The listing builds one solid part. Answer for the finished solid, in the listing's coordinates (mm). Give positions to 0.01 mm unless a question says otherwise; leave off trailing zeros. Loops run counter-clockwise (first coordinate to the right, second up) from the corner with the lowest first, then second, coordinate; pieces in that order, holes last. Notation, with made-up numbers: M 5,64.5 L 51,64.5 A20 cw 51,87.5 Z; hole C 2.5,-14.5 d4. An arc over 180 degrees is marked long. Use one line per item in the form item = value. Start each with the question number.
1. Straight lines are drawn through the part: line 1 (X direction, y = 1.45, z = 49); line 2 (X direction, y = 0.2, z = -42). For each, find the intervals that lie inside material, in ascending order. Write a range as from..to.
2. The part is cut by section C-C (z = 41.5). Write down the section's boundary in (x, y), and give its area (3 significant figures).
3. The part is cut by section A-A (y = 0.6). Give the number of separate pieces and of enclosed holes in the cut face, and give its area (3 significant figures).
4. The part is cut by section B-B (z = -44). Write down the section's boundary in (x, y), and give its area (4 significant figures).
5. The mould has two halves that part along X. Classify faces 1 (the face through (49.9, 0.7, -47.6)), 2 (the face through (-1, 1.5, -1)), 3 (the face through (-49.9, 0.7, -47.6)), 4 (the face through (-52.98, 0.76, 23.67)): released by +X, released by -X, zero draft, split by the parting line, or undercut.
from build123d import *

# Parameters (mm, degrees)
SKETCH1_W           = 115
SKETCH1_H           = 110
BOSS_EXTRUDE1_DEPTH = 1.5
CHAMFER1_SIZE       = 15
SKETCH3_R           = 1.5
CUT_EXTRUDE1_DEPTH  = 1.5
SKETCH4_R           = 1.5
CUT_EXTRUDE2_DEPTH  = 1.5


with BuildPart() as part:
    # Sketch1 → Boss-Extrude1 (new body)
    with BuildSketch(Plane(origin=(0, 0, 0), x_dir=(1, 0, 0), z_dir=(0, 1, 0))):
        Rectangle(SKETCH1_W, SKETCH1_H)
    extrude(amount=BOSS_EXTRUDE1_DEPTH)

    # Chamfer1
    chamfer1_edges = [part.edges().sort_by_distance(p)[0] for p in [
        (57.5, 0.75, 55),
        (-57.5, 0.75, 55),
        (-57.5, 0.75, -55),
        (57.5, 0.75, -55),
    ]]
    chamfer(chamfer1_edges, length=CHAMFER1_SIZE)

    # Sketch3 → Cut-Extrude1 (cut)
    with BuildSketch(Plane(origin=(0, 1.5, 0), x_dir=(1, 0, 0), z_dir=(0, 1, 0))):
        with Locations(Location((-51.515, 24, 0), (0, 0, 270))):
            Circle(SKETCH3_R)
        with Locations(Location((51.515, 24, 0), (0, 0, 270))):
            Circle(SKETCH3_R)
        with Locations(Location((51.515, -24, 0), (0, 0, 270))):
            Circle(SKETCH3_R)
        with Locations(Location((-51.515, -24, 0), (0, 0, 270))):
            Circle(SKETCH3_R)
    extrude(amount=-CUT_EXTRUDE1_DEPTH, mode=Mode.SUBTRACT)

    # Sketch4 → Cut-Extrude2 (cut)
    with BuildSketch(Plane(origin=(0, 1.5, 0), x_dir=(1, 0, 0), z_dir=(0, 1, 0))):
        with Locations(Location((-42.5, 22.5, 0), (0, 0, 270))):
            Circle(SKETCH4_R)
        with Locations(Location((-42.5, -22.5, 0), (0, 0, 270))):
            Circle(SKETCH4_R)
        with Locations(Location((42.5, -22.5, 0), (0, 0, 270))):
            Circle(SKETCH4_R)
        with Locations(Location((42.5, 22.5, 0), (0, 0, 270))):
            Circle(SKETCH4_R)
    extrude(amount=-CUT_EXTRUDE2_DEPTH, mode=Mode.SUBTRACT)


solid = part.part
Derived:
q1.line_1 = -48.5..48.5
q1.line_2 = -55.5..55.5
q2.outline = M -56,0 L 56,0 L 56,1.5 L -56,1.5 Z
q2.area = 168 mm2
q3.separate_pieces = 1
q3.enclosed_holes = 8
q3.area = 12,100 mm2
q4.outline = M -53.5,0 L 53.5,0 L 53.5,1.5 L -53.5,1.5 Z
q4.area = 160.5 mm2
q5.face_1 = released by +X
q5.face_2 = zero draft
q5.face_3 = released by -X
q5.face_4 = undercut
